Check sheet for the modelled part. Datum: model origin and axes. Units: mm. A direction names the side the tool comes from. Give positions to 0.01 mm unless a question says otherwise; leave off trailing zeros. Write each loop counter-clockwise with the first axis right and the second up, starting at its lowest first coordinate (ties: lowest second). Pieces come first, ordered by that corner, then holes. Notation, with made-up numbers: (22.5, -13) - (64.5, -13) arc R17 ccw to (64.5, 7) - close; hole circle Ø9 at (24, -20). An arc over 180 degrees is marked (long way). Return JSON: item names as keys, results as strings. Group by question number.
```python
from build123d import *

# Parameters (mm, degrees)
CUT_EXTRUDE1_DEPTH      = 18.850600229
CUT_EXTRUDE1_DEPTH_BACK = 18.850600229
SKETCH2_R               = 1.5


with BuildPart() as part:
    # Sketch1 → Revolve1 (revolve)
    with BuildSketch(Plane(origin=(0, 0, 0), x_dir=(0, 0, -1), z_dir=(1, 0, 0)), mode=Mode.PRIVATE) as revolve1_sk:
        Polygon((0, 14.85408794), (-6.25, 14.85408794), (-6.25, 13.85408794), (-7, 13.85408794), (-7, 0), (-6.2, 0), (-4.75, 3.983842258), (-4.75, 11), (0, 13.85408794), align=None)
    revolve(revolve1_sk.sketch.rotate(Axis((0, 0, 0), (0, 1, 0)), 180), axis=Axis((0, 0, 0), (0, 1, 0)))

    # Sketch2 → Cut-Extrude1 (cut, two sides: drawn at the far end of the back side and taken through both)
    with BuildSketch(Plane.XY.offset(-CUT_EXTRUDE1_DEPTH_BACK)):
        with Locations((0, 7)):
            Circle(SKETCH2_R)
    extrude(amount=CUT_EXTRUDE1_DEPTH + CUT_EXTRUDE1_DEPTH_BACK, mode=Mode.SUBTRACT)


solid = part.part
```
Item 1: Material ranges on line 1 along X through (y, z) = (5.5, 0); line 2 along X through (y, z) = (7, -6.25); line 3 along Z through (x, y) = (0.5, 2.5), recorded low to high. Write a range as from..to.
Item 2: Section check D-D on y = 7.5. Record the cut outline in (x, z), plus the area to 3 significant figures.
Item 3: Mould release check, pull along X, two halves, no side actions. Record for faces 3 (the face through (1.819, 7.541, -4.388)), 4 (the face through (-1.88, 14.35, -5.96)), 5 (the face through (5, 0, 4)): +X half, -X half, draft (parallel to the pull), parting line (faces both ways), or undercut.
Item 4: Section check C-C on x = -1. Count the separate pieces of the cut face and the enclosed holes in it, plus the area to 3 significant figures.
Item 5: Access from +Z, -Z, +X, -X, +Y, -Y to the whole of each face (thin tool, end or side, straight path). Record for faces 1 (the face through (-6, 13.854, -3)), 2 (the face through (0.74, 13.4, 0.16)).
Item 6: Section check A-A on y = 6. Record the cut outline in (x, z).
Item 7: Depth check by flat-ended pin: pin 1 (2 mm diameter, centred on y = 2.5, z = -4, fed in from +X); pin 2 (5 mm diameter, centred on x = 5, z = -2, fed in from -Y); pin 3 (3 mm diameter, centred on y = 4.5, z = 3.5, fed in from +X). Enter the tip coordinate at first touch or a pass-through.
Item 8: Section check B-B on y = 9.75. Record the cut outline in (x, z).
Reply:
{
 "1": {"line 1": "-7..-4.75, 4.75..7", "line 2": "-3.15..-1.5, 1.5..3.15", "line 3": "-6.98..-5.27, 5.27..6.98"},
 "2": {"outline": "(-1.41, -6.86) - (-1.41, -4.53) arc R4.75 cw to (-1.41, 4.53) - (-1.41, 6.86) arc R7 ccw to start; (1.41, -6.86) arc R7 ccw to (1.41, 6.86) - (1.41, 4.53) arc R4.75 cw to (1.41, -4.53) - close", "area": "70.2 mm²"},
 "3": {"face 3": "undercut", "face 4": "parting line", "face 5": "draft"},
 "4": {"separate pieces": "3", "enclosed holes": "0", "area": "74.1 mm²"},
 "5": {"face 1": "+Y", "face 2": "-Y"},
 "6": {"outline": "(-1.12, -6.91) - (-1.12, -4.62) arc R4.75 cw to (-1.12, 4.62) - (-1.12, 6.91) arc R7 ccw to start; (1.12, -6.91) arc R7 ccw to (1.12, 6.91) - (1.12, 4.62) arc R4.75 cw to (1.12, -4.62) - close"},
 "7": {"pin 1": "x = 6.32", "pin 2": "y = 0", "pin 3": "x = 6.71"},
 "8": {"outline": "circle Ø14 at (0, 0); hole circle Ø9.5 at (0, 0)"}
}
